Can you work these out from the model? Positions are in its coordinate system, mm. A direction names the side the tool comes from. Coordinates: 2 decimals unless noted, no trailing zeros. Loops run counter-clockwise (first coordinate to the right, second up) from the corner with the lowest first, then second, coordinate; pieces in that order, holes last.
```python
from build123d import *

# Parameters (mm, degrees)
SKETCH1_R           = 4.7625
SKETCH1_R_2         = 2
BOSS_EXTRUDE2_DEPTH = 12.7
SKETCH2_R           = 2
CUT_EXTRUDE1_DEPTH  = 2.5


with BuildPart() as part:
    # Sketch1 → Boss-Extrude2 (new body)
    with BuildSketch(Plane.XY):
        with BuildLine():
            Line((0, 21), (100, 21))
            ThreePointArc((100, 21), (121, 0), (100, -21))
            Line((100, -21), (0, -21))
            ThreePointArc((0, -21), (-21, 0), (0, 21))
        make_face()
        with Locations((100, 0)):
            Circle(SKETCH1_R, mode=Mode.SUBTRACT)
        with Locations((15, 0)):
            Circle(SKETCH1_R_2, mode=Mode.SUBTRACT)
        with Locations((-7.5, -12.990381057)):
            Circle(SKETCH1_R_2, mode=Mode.SUBTRACT)
        with Locations((-7.5, 12.990381057)):
            Circle(SKETCH1_R_2, mode=Mode.SUBTRACT)
    extrude(amount=BOSS_EXTRUDE2_DEPTH)

    # Sketch2 → Cut-Extrude1 (cut)
    with BuildSketch(Plane.XY.offset(12.7)):
        with Locations((-13.5, 0)):
            Circle(SKETCH2_R)
        with Locations((6.75, 11.691342951)):
            Circle(SKETCH2_R)
        with Locations((6.75, -11.691342951)):
            Circle(SKETCH2_R)
    extrude(amount=-CUT_EXTRUDE1_DEPTH, mode=Mode.SUBTRACT)


solid = part.part
```
Item 1: I need wall thicknesses on line 1 along X through (y, z) = (-1.5, 7.5); line 2 along X through (y, z) = (-14, 9.75); line 3 along X through (y, z) = (12.5, 5). Which ranges of each line are inside material? Lowest first, please.
Results are:
line 1: x = -20.95 to 13.68, 16.32 to 95.48, 104.52 to 120.95
line 2: x = -15.65 to -9.23, -5.77 to 115.65
line 3: x = -16.87 to -9.44, -5.56 to 116.87
Item 2: Suppose I cut it at C-C, the plane z = 6.75. Please give me the cut outline in (x, y) (1 decimal), plus the area to 3 significant figures.
Results are:
outline: (0, -21) - (100, -21) arc R21 ccw to (100, 21) - (0, 21) arc R21 ccw to start; hole circle Ø4 at (-7.5, -13); hole circle Ø4 at (-7.5, 13); hole circle Ø4 at (15, 0); hole circle Ø9.5 at (100, 0)
area: 5,480 mm2
Item 3: We'd pull the mould along X, two halves only. Please class faces 1 (the face through (121, 0, 6)), 2 (the face through (51, 0, 0)), 3 (the face through (-15.1, -1.2, 11.5)): +X half, -X half, draft (parallel to the pull), parting line (faces both ways), or undercut.
Results are:
face 1: +X half
face 2: draft
face 3: undercut
Item 4: Suppose I cut it at A-A, the plane x = 15. Please give me the cut outline in (y, z), plus the area to 3 significant figures.
Results are:
outline: (-21, 0) - (-2, 0) - (-2, 12.7) - (-21, 12.7) - close; (2, 0) - (21, 0) - (21, 12.7) - (2, 12.7) - close
area: 483 mm2
Item 5: On a 3-axis mill with a long thin cutter (end or side, diameter ignored), from which of +Z, -Z, +X, -X, +Y, -Y can I reach the whole of each face in a straight line? I mean faces 4 (the face through (7, -12, 10.2)), 5 (the face through (95.242, 0.209, 6.261)). Say none if no direction works.
Results are:
face 4: +Z
face 5: +Z, -Z
Item 6: I'm going to push flat-ended pins straight in: P1, Ø2, axis at x = 6.5, y = 12, coming from the +Z side; P2, Ø6.5, axis at x = -7.5, y = -12.99, coming from the -Z side; P3, Ø2, axis at y = 2.5, z = 3.5, coming from the +X side; P4, Ø1, axis at y = -4, z = 3.5, coming from the +X side. Where does each tip first touch, or does it pass through?
Results are:
P1: stops at z = 10.2
P2: stops at z = 0
P3: stops at x = 120.95
P4: stops at x = 120.71
Item 7: Suppose I cut it at D-D, the plane x = -13.5. Please give me the cut outline in (y, z), plus the area to 3 significant figures.
Results are:
outline: (-16.09, 0) - (16.09, 0) - (16.09, 12.7) - (2, 12.7) - (2, 10.2) - (-2, 10.2) - (-2, 12.7) - (-16.09, 12.7) - close
area: 399 mm2
Item 8: Suppose I cut it at B-B, the plane y = 0. Please give me the cut outline in (x, z), plus the area to 3 significant figures.
Results are:
outline: (-21, 0) - (13, 0) - (13, 12.7) - (-11.5, 12.7) - (-11.5, 10.2) - (-15.5, 10.2) - (-15.5, 12.7) - (-21, 12.7) - close; (17, 0) - (95.24, 0) - (95.24, 12.7) - (17, 12.7) - close; (104.76, 0) - (121, 0) - (121, 12.7) - (104.76, 12.7) - close
area: 1,620 mm2
